Input: part model. Units: mm. Frame: model coordinates. Face numbers are marked on the shaded views. A direction names the side the tool comes from. Round coordinates to 2 decimals unless told otherwise and drop trailing zeros. Write each loop counter-clockwise with the first axis right and the second up, starting at its lowest first coordinate (ties: lowest second). Pieces come first, ordered by that corner, then holes. Notation, with made-up numbers: (-16.75, -32) - (20.25, -32) arc R24 cw to (20.25, -11) - close; hole circle Ø4 at (80.25, -34). An arc over 180 degrees is marked (long way). One line per item, written item: value. Start each with the question number.
```python
from build123d import *

# Parameters (mm, degrees)
F1_DEPTH      = 500
F1_DEPTH_BACK = 500
F3_DEPTH      = 150
F5_DEPTH      = 840


with BuildPart() as f1:
    # F0 (on Right) → F1 (new body, two sides)
    with BuildSketch(Plane.YZ) as f1_sk:
        Polygon((-1780, 0), (0, 0), (0, 860), (-377.893543, 860), (-377.893543, 679.984152), (-727.893543, 679.984152), (-727.893543, 499.984152), (-1077.893543, 499.984152), (-1077.893543, 319.984152), (-1427.893543, 319.984152), (-1427.893543, 139.984152), (-1777.893543, 139.984152), align=None)
    extrude(amount=F1_DEPTH)
    extrude(f1_sk.sketch, amount=-F1_DEPTH_BACK)

    # F2 (on face) → F3 (join)
    with BuildSketch(Plane.YZ.offset(500)):
        Polygon((0, 860), (-377.893543, 860), (-1777.893543, 139.984152), (-1780, 0), (0, 0), align=None)
    extrude(amount=F3_DEPTH)

    # F4 (on face) → F5 (join)
    with BuildSketch(Plane(origin=(-500, 0, 0), x_dir=(0, -1, 0), z_dir=(-1, 0, 0))):
        Polygon((1780, 0), (1777.893543, 139.984152), (377.893543, 860), (0, 860), (0, 0), align=None)
    extrude(amount=F5_DEPTH)


solid = f1.part
```
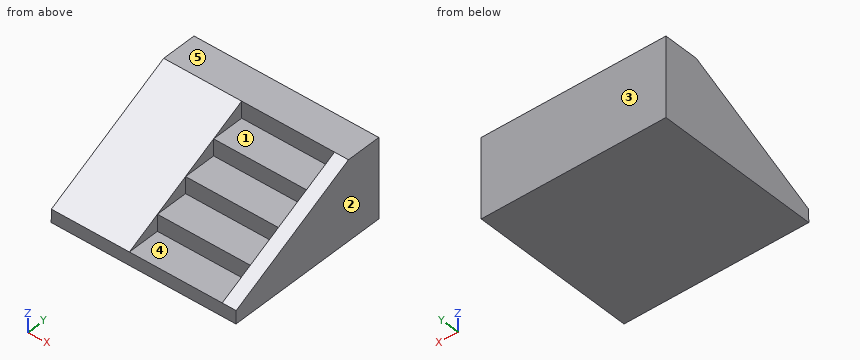
Q1. Cut plane D-D, the plane x = 257.5. Output: boundary loops of the cut face in (y, z), and give its area (3 significant figures).
Q2. Cut plane A-A, the plane x = -544. Output: boundary loops of the cut face in (y, z), and give its area (3 significant figures).
Q3. Access query for the marked faces 4 and 5. Directions: +Z, -Z, +X, -X, +Y, -Y. A direction counts if a zero-diameter tool reaches every point of the face in a straight line with its end or side. Return the directions, or none.
Q4. Cut plane B-B, the plane z = 762.5. Output: boundary loops of the cut face in (x, y).
Q5. Pull-direction query (X, two-part tool) for the marked faces 1, 2 and 3; classes: pulls with the +X half, pulls with the -X half, needs draft (parallel to the pull), parting line crosses it, or undercut.
Q6. Cut plane C-C, the plane y = -960.5. Output: boundary loops of the cut face in (x, z), and give its area (3 significant figures).
Q7. Material intervals for probe 1 along X at (y, z) = (-795.5, 589); probe 2 along Y at (x, z) = (-791, 114); probe 3 along Y at (x, z) = (-320, 313), sorted ascending. Write a range as from..to.
Q8. Contact query for flat-ended pins moving along their axis: pin 1 Ø1.5 at (x, y) = (-447, -945.5) entering from +Z; pin 2 Ø3 at (x, y) = (51.5, -1243) entering from -Z; pin 3 Ø2 at (x, z) = (-436, 489) entering from -Y. Output: stop coordinate, or through.
A:
1. outline: (-1780, 0) - (0, 0) - (0, 860) - (-377.89, 860) - (-377.89, 679.98) - (-727.89, 679.98) - (-727.89, 499.98) - (-1077.89, 499.98) - (-1077.89, 319.98) - (-1427.89, 319.98) - (-1427.89, 139.98) - (-1777.89, 139.98) - close
1. area: 899,000 mm²
2. outline: (-1780, 0) - (0, 0) - (0, 860) - (-377.89, 860) - (-1777.89, 139.98) - close
2. area: 1,030,000 mm²
3. face 4: +Z, -Y
3. face 5: +Z, +X, -X, +Y, -Y
4. outline: (-1340, -567.47) - (-500, -567.47) - (-500, -377.89) - (500, -377.89) - (500, -567.47) - (650, -567.47) - (650, 0) - (-1340, 0) - close
5. face 1: undercut
5. face 2: pulls with the +X half
5. face 3: needs draft
6. outline: (-1340, 0) - (650, 0) - (650, 560.37) - (500, 560.37) - (500, 499.98) - (-500, 499.98) - (-500, 560.37) - (-1340, 560.37) - close
6. area: 1,050,000 mm²
7. probe 1: x = -1340..-500, 500..650
7. probe 2: y = -1778.28..0
7. probe 3: y = -1427.89..0
8. pin 1: stops at z = 499.98
8. pin 2: stops at z = 0
8. pin 3: stops at y = -1077.89
